Check sheet for the modelled part. Datum: model origin and axes. Units: mm. A direction names the side the tool comes from. Give positions to 0.01 mm unless a question says otherwise; leave off trailing zeros. Loops run counter-clockwise (first coordinate to the right, second up) from the corner with the lowest first, then second, coordinate; pieces in that order, holes last. Notation, with made-up numbers: (-12, 5) - (8, 5) arc R22 ccw to (8, 29) - close; hole circle Ø7 at (-30.75, -28). An arc over 180 degrees is marked (long way). Answer in a Markdown table with one row per item. Add a question column.
(1) Sectioned sample at A-A on y = 107.5. Enter the section's corners in (x, z), then the cut area to 3 significant figures.
(2) Thickness scan on L1, parallel to Y at x = 47.5, z = 1.5; L2, parallel to X at y = 28, z = -0.5; L3, parallel to Y at x = -72, z = 3. Record the ranges inside material, lowest first.
(3) Draft check along X on faces 1 (the face through (9.216, 6.568, -0.083)), 2 (the face through (4, 48, -4.762)), 3 (the face through (25.21, 82.7, -0.07)). Enter one of: released by +X, released by -X, zero draft, split by the parting line, or undercut.
(4) Sectioned sample at B-B on x = 7. Enter the section's corners in (y, z).
(5) Set-up check for faces 4 (the face through (-44.76, 6.57, -0.08)), 5 (the face through (70, 120.65, 0)), 6 (the face through (59, 110.998, 0)): record each of +Z, -Z, +X, -X, +Y, -Y from which the full face is reachable in a straight line by a thin tool's end or side.
(6) Go/stop test with flat-tipped pins: P1, Ø3, axis at x = 58.54, z = 0, coming from the -Y side; P2, Ø1.1, axis at x = 80.5, z = -1, coming from the +Y side; P3, Ø1, axis at y = 80.5, z = 0, coming from the -X side. Record where each tip stops, or that it passes through.
from build123d import *

# Parameters (mm, degrees)
SKETCH1_W                  = 44.45
SKETCH1_H                  = 9.525
F_10_24_TAPPED_HOLE1_D     = 3.7973
F_10_24_TAPPED_HOLE1_DEPTH = 12.954
F_10_24_TAPPED_HOLE2_D     = 3.7973
F_10_24_TAPPED_HOLE2_DEPTH = 9.652
BOSS_EXTRUDE1_DEPTH        = 9.525
F_10_24_TAPPED_HOLE3_D     = 3.7973
F_10_24_TAPPED_HOLE3_DEPTH = 12.954
F_10_24_TAPPED_HOLE3_TIP   = 1.140824014
FILLET1_R                  = 12.7


with BuildPart() as part:
    # Sweep1: sweep along a path in Sketch2
    with BuildLine(Plane.XY) as sweep1_path:
        Line((-22.225, 0), (47.432309978, 120.65))
    # Sketch1 → Sweep1 (sweep)
    with BuildSketch(Plane(origin=(0, 0, 0), x_dir=(1, 0, 0), z_dir=(0, 1, 0))):
        Rectangle(SKETCH1_W, SKETCH1_H)
    sweep(path=sweep1_path.line)

    # #10-24 Tapped Hole1
    with Locations(Plane(origin=(0, 0, 0), x_dir=(-1, 0, 0), z_dir=(0, -1, 0))):
        with Locations((11.1125, 0), (-11.1125, 0)):
            Hole(F_10_24_TAPPED_HOLE1_D / 2, depth=F_10_24_TAPPED_HOLE1_DEPTH)

    # #10-24 Tapped Hole2
    with Locations(Plane(origin=(0, 120.65, 0), x_dir=(1, 0, 0), z_dir=(0, 1, 0))):
        with Locations((58.544809978, 0), (80.769809978, 0)):
            Hole(F_10_24_TAPPED_HOLE2_D / 2, depth=F_10_24_TAPPED_HOLE2_DEPTH)

    # Sketch14 → Boss-Extrude1 (add)
    with BuildSketch(Plane.XY.offset(4.7625)):
        Polygon((-22.225, 0), (-85.725, 0), (25.435264722, 82.55), align=None)
    extrude(amount=-BOSS_EXTRUDE1_DEPTH)

    # #10-24 Tapped Hole3
    with Locations(Plane(origin=(0, 0, 0), x_dir=(-1, 0, 0), z_dir=(0, -1, 0))):
        with Locations((42.8625, 0), (65.0875, 0)):
            Hole(F_10_24_TAPPED_HOLE3_D / 2, depth=F_10_24_TAPPED_HOLE3_DEPTH)
            with Locations((0, 0, -(F_10_24_TAPPED_HOLE3_DEPTH + F_10_24_TAPPED_HOLE3_TIP / 2))):  # 118° drill point
                Cone(0, F_10_24_TAPPED_HOLE3_D / 2, F_10_24_TAPPED_HOLE3_TIP, mode=Mode.SUBTRACT)

    # Fillet1
    fillet1_edges = [part.edges().sort_by_distance(p)[0] for p in [
        (25.435264722, 82.55, 0),
    ]]
    fillet(fillet1_edges, radius=FILLET1_R)


solid = part.part
Reply:
| question | item | result |
|---|---|---|
| 1 | outline | (39.84, -4.76) - (84.29, -4.76) - (84.29, 4.76) - (39.84, 4.76) - close |
| 1 | area | 423 mm^2 |
| 2 | L1 | 43.78 to 120.65 |
| 2 | L2 | -48.02 to 38.39 |
| 2 | L3 | 0 to 10.19 |
| 3 | face 1 | undercut |
| 3 | face 2 | zero draft |
| 3 | face 3 | released by -X |
| 4 | outline | (0, -4.76) - (68.86, -4.76) - (68.86, 4.76) - (0, 4.76) - close |
| 5 | face 4 | -Y |
| 5 | face 5 | +Z, -Z, +X, -X, +Y |
| 5 | face 6 | +Y |
| 6 | P1 | y = 60.3 |
| 6 | P2 | y = 111 |
| 6 | P3 | x = 22 |
